Check sheet for the modelled part. Datum: model origin and axes. Units: mm. A direction names the side the tool comes from. Round coordinates to 2 decimals unless told otherwise and drop trailing zeros. Order: outer loops, then holes, each group sorted by start corner. A loop starts at its lowest first (then second) coordinate and runs counter-clockwise, first axis right, second up. Notation, with made-up numbers: (39, -37) -> (79, -37) arc R24 ccw to (79, -20) -> close; hole circle Ø10 at (-20, 73.25). An arc over 180 degrees is marked (long way). Answer in a Markdown table with one row per item. Add a question column.
1. Material ranges on L1, parallel to Y at x = 37.36, z = 1.85; L2, parallel to Y at x = 27.64, z = 0.9; L3, parallel to Y at x = -37, z = 0.3, recorded low to high. Write a range as from..to.
2. Sectioned sample at A-A, the plane x = -28. Record the boundary of the cut face in (y, z), then the cut area to 3 significant figures.
3. Depth check by flat-ended pin: P1, Ø2, axis at x = 30, y = -5.5, coming from the -Z side; P2, Ø0.6, axis at x = 45.5, z = -1.5, coming from the -Y side. Enter the tip coordinate at first touch or a pass-through.
4. Sectioned sample at B-B, the plane x = 16.5. Record the boundary of the cut face in (y, z).
5. Sectioned sample at C-C, the plane y = -4. Record the boundary of the cut face in (x, z).
6. Access from +Z, -Z, +X, -X, +Y, -Y to the whole of each face (thin tool, end or side, straight path). Record for faces 1 (the cylindrical face through (35.73, 20.09, 1.48)), 2 (the flat face through (46, 3, -1.5)), 3 (the flat face through (-26, -5, 0.5)).
7. Draft check along Y on faces 4 (the flat face through (-1, -50, 1)), 5 (the flat face through (46, -16, -1.5)), 6 (the flat face through (7, -27, 0.5)). Enter one of: +Y half, -Y half, draft (parallel to the pull), parting line (faces both ways), or undercut.
8. Sectioned sample at D-D, the plane z = 1.35. Count the separate pieces of the cut face and the enclosed holes in it, then the cut area to 3 significant figures.
```python
from build123d import *

# Parameters (mm, degrees)
SKETCH_W        = 100
SKETCH_H        = 100
SKETCH_R        = 1.5
SKETCH_R_2      = 2.75
PAD_DEPTH       = 3
SKETCH001_W     = 14
SKETCH001_H     = 9.2
SKETCH001_W_2   = 10.3
SKETCH001_H_2   = 20.6
SKETCH001_W_3   = 36.2
SKETCH001_H_3   = 10.3
POCKET_DEPTH    = 0.5
SKETCH002_W     = 6.3
SKETCH002_H     = 5.4
PAD001_DEPTH    = 2
SKETCH003_W     = 5.3
SKETCH003_H     = 5.4
POCKET001_DEPTH = 0.5


with BuildPart() as part:
    # Sketch → Pad (new body)
    with BuildSketch(Plane.XY):
        Rectangle(SKETCH_W, SKETCH_H)
        with Locations((-44, 44)):
            Circle(SKETCH_R, mode=Mode.SUBTRACT)
        with Locations((44, 44)):
            Circle(SKETCH_R, mode=Mode.SUBTRACT)
        with Locations((44, -44)):
            Circle(SKETCH_R, mode=Mode.SUBTRACT)
        with Locations((-44, -44)):
            Circle(SKETCH_R, mode=Mode.SUBTRACT)
        with Locations((-43.3, 19.64)):
            Circle(SKETCH_R, mode=Mode.SUBTRACT)
        with Locations((-34.3, 19.64)):
            Circle(SKETCH_R, mode=Mode.SUBTRACT)
        with Locations((16.3, 19.64)):
            Circle(SKETCH_R, mode=Mode.SUBTRACT)
        with Locations((25.3, 19.64)):
            Circle(SKETCH_R, mode=Mode.SUBTRACT)
        with Locations((34.3, 19.64)):
            Circle(SKETCH_R, mode=Mode.SUBTRACT)
        with Locations((43.3, 19.64)):
            Circle(SKETCH_R, mode=Mode.SUBTRACT)
        with Locations((-25.3, 19.64)):
            Circle(SKETCH_R, mode=Mode.SUBTRACT)
        with Locations((-16.3, 19.64)):
            Circle(SKETCH_R, mode=Mode.SUBTRACT)
        with Locations((-37.6, -43)):
            Circle(SKETCH_R_2, mode=Mode.SUBTRACT)
        with Locations((-27.6, -43)):
            Circle(SKETCH_R_2, mode=Mode.SUBTRACT)
        with Locations((-17.6, -43)):
            Circle(SKETCH_R_2, mode=Mode.SUBTRACT)
        with Locations((-7.6, -43)):
            Circle(SKETCH_R_2, mode=Mode.SUBTRACT)
        with Locations((7.64, -43)):
            Circle(SKETCH_R_2, mode=Mode.SUBTRACT)
        with Locations((27.64, -43)):
            Circle(SKETCH_R_2, mode=Mode.SUBTRACT)
        with Locations((37.64, -43)):
            Circle(SKETCH_R_2, mode=Mode.SUBTRACT)
        with Locations((17.64, -43)):
            Circle(SKETCH_R_2, mode=Mode.SUBTRACT)
        with Locations((37.36, 44.6)):
            Circle(SKETCH_R_2, mode=Mode.SUBTRACT)
        with Locations((37.34, -30.60363)):
            Circle(SKETCH_R_2, mode=Mode.SUBTRACT)
        with Locations((17.34, -30.60363)):
            Circle(SKETCH_R_2, mode=Mode.SUBTRACT)
    extrude(amount=PAD_DEPTH)

    # Sketch001 (on Face28 of Pad) → Pocket (cut)
    with BuildSketch(Plane(origin=(0, 0, 0), x_dir=(1, 0, 0), z_dir=(0, 0, -1))):
        with Locations((-42.6, 30.5)):
            Rectangle(SKETCH001_W, SKETCH001_H)
        with Locations((-11.35, 26.87)):
            Rectangle(SKETCH001_W_2, SKETCH001_H_2)
        with Locations((7.33, 26.87)):
            Rectangle(SKETCH001_W_2, SKETCH001_H_2)
        with Locations((27.33, 26.87)):
            Rectangle(SKETCH001_W_2, SKETCH001_H_2)
        with Locations((-25.9, 5)):
            Rectangle(SKETCH001_W_3, SKETCH001_H_3)
    extrude(amount=-POCKET_DEPTH, mode=Mode.SUBTRACT)

    # Sketch002 (on Face4 of Pocket) → Pad001 (join)
    with BuildSketch(Plane(origin=(0, 0, 0), x_dir=(1, 0, 0), z_dir=(0, 0, -1))):
        with Locations((46.85, -3.3)):
            Rectangle(SKETCH002_W, SKETCH002_H)
        with Locations((46.85, 3.24)):
            Rectangle(SKETCH002_W, SKETCH002_H)
        with Locations((46.85, 9.78)):
            Rectangle(SKETCH002_W, SKETCH002_H)
        with Locations((46.85, 16.32)):
            Rectangle(SKETCH002_W, SKETCH002_H)
    extrude(amount=PAD001_DEPTH)

    # Sketch003 (on Face61 of Pad001) → Pocket001 (cut)
    with BuildSketch(Plane(origin=(0, 0, -2), x_dir=(1, 0, 0), z_dir=(0, 0, -1))):
        with Locations((46.35, -3.3)):
            Rectangle(SKETCH003_W, SKETCH003_H)
        with Locations((46.35, 3.24)):
            Rectangle(SKETCH003_W, SKETCH003_H)
        with Locations((46.35, 9.78)):
            Rectangle(SKETCH003_W, SKETCH003_H)
        with Locations((46.35, 16.32)):
            Rectangle(SKETCH003_W, SKETCH003_H)
    extrude(amount=-POCKET001_DEPTH, mode=Mode.SUBTRACT)


solid = part.part
```
Answer key:
| question | item | result |
|---|---|---|
| 1 | L1 | y = -50..-45.74, -40.26..-33.35, -27.85..41.85, 47.35..50 |
| 1 | L2 | y = -50..-45.75, -40.25..50 |
| 1 | L3 | y = -50..-45.68, -40.32..-35.1, -25.9..-10.15, 0.15..50 |
| 2 | outline | (-50, 0) -> (-45.72, 0) -> (-45.72, 3) -> (-50, 3) -> close; (-40.28, 0) -> (-10.15, 0) -> (-10.15, 0.5) -> (0.15, 0.5) -> (0.15, 0) -> (50, 0) -> (50, 3) -> (-40.28, 3) -> close |
| 2 | area | 279 mm² |
| 3 | P1 | stops at z = 0 |
| 3 | P2 | stops at y = -19.02 |
| 4 | outline | (-50, 0) -> (-45.5, 0) -> (-45.5, 3) -> (-50, 3) -> close; (-40.5, 0) -> (-33.22, 0) -> (-33.22, 3) -> (-40.5, 3) -> close; (-27.99, 0) -> (18.15, 0) -> (18.15, 3) -> (-27.99, 3) -> close; (21.13, 0) -> (50, 0) -> (50, 3) -> (21.13, 3) -> close |
| 5 | outline | (-50, 0) -> (-44, 0) -> (-44, 0.5) -> (-7.8, 0.5) -> (-7.8, 0) -> (43.7, 0) -> (43.7, -1.5) -> (49, -1.5) -> (49, -2) -> (50, -2) -> (50, 3) -> (-50, 3) -> close |
| 6 | face 1 | +Z, -Z |
| 6 | face 2 | -Z, -X, +Y, -Y |
| 6 | face 3 | -Z |
| 7 | face 4 | -Y half |
| 7 | face 5 | draft |
| 7 | face 6 | undercut |
| 8 | separate pieces | 1 |
| 8 | enclosed holes | 23 |
| 8 | area | 9,650 mm² |
